from build123d import *

# Parameters (mm, degrees)
EXTRUDE_3_DEPTH     = 70
CUT_EXTRUDE_2_DEPTH = 5
CUT_EXTRUDE_4_DEPTH = 35


with BuildPart() as part:
    # 草图1 → 凸台-拉伸3 (new body)
    with BuildSketch(Plane.XY):
        with BuildLine():
            Line((48, 36), (48, -36))
            ThreePointArc((48, -36), (-60, 0), (48, 36))
        make_face()
    extrude(amount=EXTRUDE_3_DEPTH)

    # 草图4 → 切除-拉伸2 (cut)
    with BuildSketch(Plane(origin=(48, 0, 0), x_dir=(0, 0, -1), z_dir=(1, 0, 0))):
        Polygon((-28.839745962, -3.556624327), (-28.839745962, -6.443375673), (-26.339745962, -7.886751346), (-23.839745962, -6.443375673), (-23.839745962, -3.556624327), (-26.339745962, -2.113248654), align=None)
        Polygon((-35, 7.113248654), (-32.5, 8.556624327), (-32.5, 11.443375673), (-35, 12.886751346), (-37.5, 11.443375673), (-37.5, 8.556624327), align=None)
        Polygon((-41.160254038, -3.556624327), (-43.660254038, -2.113248654), (-46.160254038, -3.556624327), (-46.160254038, -6.443375673), (-43.660254038, -7.886751346), (-41.160254038, -6.443375673), align=None)
    extrude(amount=-CUT_EXTRUDE_2_DEPTH, mode=Mode.SUBTRACT)

    # 草图6 → 切除-拉伸4 (cut)
    with BuildSketch(Plane.XY.offset(70)):
        with BuildLine():
            Line((42.4984665, 38.306424351), (42.4984665, -38.306424351))
            ThreePointArc((42.4984665, -38.306424351), (-57.214524392, 0), (42.4984665, 38.306424351))
        make_face()
    extrude(amount=-CUT_EXTRUDE_4_DEPTH, mode=Mode.SUBTRACT)


solid = part.part
Input: part model. Units: mm. Frame: model coordinates. A direction names the side the tool comes from. Coordinates: 2 decimals unless noted, no trailing zeros. Write each loop counter-clockwise with the first axis right and the second up, starting at its lowest first coordinate (ties: lowest second). Pieces come first, ordered by that corner, then holes. Notation, with made-up numbers: M 46.5,59.25 L 86.5,59.25 A19 cw 86.5,86.25 Z; hole C 49,-21 d11. An arc over 180 degrees is marked long. Answer as a JSON object with one key per item and string values. Group by question number.
(1) Set-up query: faces 1 (the face through (-5, 1, 0)), 2 (the face through (-7, 1, 35)), 3 (the face through (46, -5, 23.84)). Return all of +Z, -Z, +X, -X, +Y, -Y with unobstructed straight access to the full face (end or side cutting, diameter ignored); none if empty.
(2) Contact query for flat-ended pins moving along their axis: P1, Ø6, axis at x = 17.5, y = -45, coming from the +Z side; P2, Ø1.5, axis at y = 11, z = 35, coming from the +X side; P3, Ø6, axis at x = -34, z = 33, coming from the -Y side. Output: stop coordinate, or through.
(3) Section A-A on x = 0. Output: boundary loops of the cut face in (y, z), plus the area to 3 significant figures.
(4) Mould query, pull axis X, two halves, no side actions, for faces 4 (the face through (-57.18, -1.93, 52.74)), 5 (the face through (42.498, 1, 53)), 6 (the face through (46, -5, 28.84)), 7 (the face through (48, 1, 35)). Classes: pulls with the +X half, pulls with the -X half, needs draft (parallel to the pull), parting line crosses it, or undercut.
(5) Ray query, line 1 along Y through (x, z) = (0, 49); line 2 along X through (y, z) = (0, 49); line 3 along Z through (x, y) = (32, -18). Return the intervals inside material, ascending. Write a range as [from, to].
(6) Section C-C on z = 18. Output: boundary loops of the cut face in (x, y), plus the area to 3 significant figures.
(7) Section B-B on y = 0. Output: boundary loops of the cut face in (x, z).
Result set:
{
 "1": {"face 1": "-Z, +X, -X, +Y, -Y", "face 2": "+Z", "face 3": "+X"},
 "2": {"P1": "stops at z = 35", "P2": "stops at x = 43", "P3": "stops at y = -51.37"},
 "3": {"outline": "M -60,0 L 60,0 L 60,70 L 57.21,70 L 57.21,35 L -57.21,35 L -57.21,70 L -60,70 Z", "area": "4,390 mm2"},
 "4": {"face 4": "undercut", "face 5": "undercut", "face 6": "needs draft", "face 7": "pulls with the +X half"},
 "5": {"line 1": "y = [-60, -57.21], [57.21, 60]", "line 2": "x = [-60, -57.21], [42.5, 48]", "line 3": "z = [0, 35]"},
 "6": {"outline": "M 48,-36 L 48,36 A60 ccw long Z", "area": "10,700 mm2"},
 "7": {"outline": "M -60,0 L 48,0 L 48,70 L 42.5,70 L 42.5,35 L -57.21,35 L -57.21,70 L -60,70 Z"}
}
